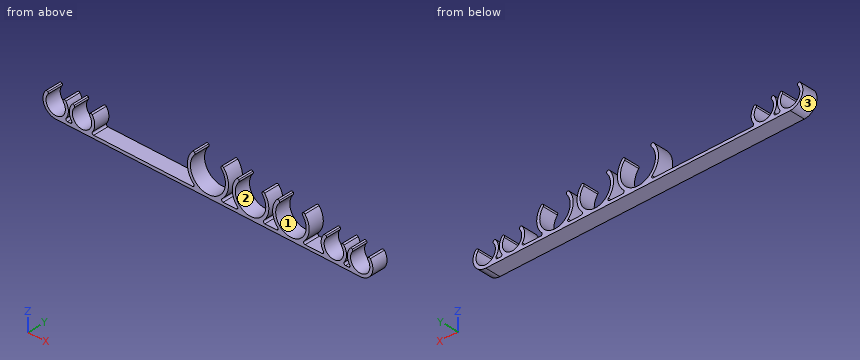
```python
from build123d import *

# Parameters (mm, degrees)
F1_DEPTH = 10


with BuildPart() as f1:
    # F0 (on Front) → F1 (new body)
    with BuildSketch(Plane.XZ):
        with BuildLine():
            Line((-100, 0), (0, 0))
            Line((0, 0), (100, 0))
            ThreePointArc((100, 0), (107.478558, 4.636017), (106.652751, 13.396128))
            ThreePointArc((106.652751, 13.396128), (105.9242, 13.789474), (105.148908, 13.498908))
            ThreePointArc((105.148908, 13.498908), (104.858342, 12.859987), (105.059278, 12.187474))
            ThreePointArc((105.059278, 12.187474), (100, 2), (94.940722, 12.187474))
            ThreePointArc((94.940722, 12.187474), (95.141658, 12.859987), (94.851092, 13.498908))
            ThreePointArc((94.851092, 13.498908), (94.0758, 13.789474), (93.347249, 13.396128))
            ThreePointArc((93.347249, 13.396128), (91.651649, 8.515919), (93.152004, 3.572193))
            ThreePointArc((93.152004, 3.572193), (93.218505, 2.537503), (92.331884, 2))
            Line((92.331884, 2), (90.368116, 2))
            ThreePointArc((90.368116, 2), (89.481495, 2.537503), (89.547996, 3.572193))
            ThreePointArc((89.547996, 3.572193), (91.048351, 8.515919), (89.352751, 13.396128))
            ThreePointArc((89.352751, 13.396128), (88.6242, 13.789474), (87.848908, 13.498908))
            ThreePointArc((87.848908, 13.498908), (87.558342, 12.859987), (87.759278, 12.187474))
            ThreePointArc((87.759278, 12.187474), (82.7, 2), (77.640722, 12.187474))
            ThreePointArc((77.640722, 12.187474), (77.841658, 12.859987), (77.551092, 13.498908))
            ThreePointArc((77.551092, 13.498908), (76.7758, 13.789474), (76.047249, 13.396128))
            ThreePointArc((76.047249, 13.396128), (74.351649, 8.515919), (75.852004, 3.572193))
            ThreePointArc((75.852004, 3.572193), (75.918505, 2.537503), (75.031884, 2))
            Line((75.031884, 2), (63.880832, 2))
            ThreePointArc((63.880832, 2), (62.960965, 2.607768), (63.159229, 3.692308))
            ThreePointArc((63.159229, 3.692308), (66.492584, 11.578174), (63.721535, 19.678756))
            ThreePointArc((63.721535, 19.678756), (62.998575, 20.037824), (62.245967, 19.745967))
            ThreePointArc((62.245967, 19.745967), (61.954109, 19.084362), (62.184612, 18.398964))
            ThreePointArc((62.184612, 18.398964), (54.5, 2), (46.815388, 18.398964))
            ThreePointArc((46.815388, 18.398964), (47.045891, 19.084362), (46.754033, 19.745967))
            ThreePointArc((46.754033, 19.745967), (46.001425, 20.037824), (45.278465, 19.678756))
            ThreePointArc((45.278465, 19.678756), (42.507416, 11.578174), (45.840771, 3.692308))
            ThreePointArc((45.840771, 3.692308), (46.039035, 2.607768), (45.119168, 2))
            Line((45.119168, 2), (37.380832, 2))
            ThreePointArc((37.380832, 2), (36.460965, 2.607768), (36.659229, 3.692308))
            ThreePointArc((36.659229, 3.692308), (39.992584, 11.578174), (37.221535, 19.678756))
            ThreePointArc((37.221535, 19.678756), (36.498575, 20.037824), (35.745967, 19.745967))
            ThreePointArc((35.745967, 19.745967), (35.454109, 19.084362), (35.684612, 18.398964))
            ThreePointArc((35.684612, 18.398964), (28, 2), (20.315388, 18.398964))
            ThreePointArc((20.315388, 18.398964), (20.545891, 19.084362), (20.254033, 19.745967))
            ThreePointArc((20.254033, 19.745967), (19.501425, 20.037824), (18.778465, 19.678756))
            ThreePointArc((18.778465, 19.678756), (16.007416, 11.578174), (19.340771, 3.692308))
            ThreePointArc((19.340771, 3.692308), (19.539035, 2.607768), (18.619168, 2))
            Line((18.619168, 2), (10, 2))
            ThreePointArc((10, 2), (9.071523, 2.628609), (9.310345, 3.724138))
            ThreePointArc((9.310345, 3.724138), (13.481586, 12.795141), (10.279021, 22.25167))
            ThreePointArc((10.279021, 22.25167), (9.557644, 22.602597), (8.810505, 22.310505))
            ThreePointArc((8.810505, 22.310505), (8.518413, 21.64343), (8.756203, 20.955126))
            ThreePointArc((8.756203, 20.955126), (0, 2), (-8.756203, 20.955126))
            ThreePointArc((-8.756203, 20.955126), (-8.518413, 21.64343), (-8.810505, 22.310505))
            ThreePointArc((-8.810505, 22.310505), (-9.557644, 22.602597), (-10.279021, 22.25167))
            ThreePointArc((-10.279021, 22.25167), (-13.481586, 12.795141), (-9.310345, 3.724138))
            ThreePointArc((-9.310345, 3.724138), (-9.071523, 2.628609), (-10, 2))
            Line((-10, 2), (-75.031884, 2))
            ThreePointArc((-75.031884, 2), (-75.918505, 2.537503), (-75.852004, 3.572193))
            ThreePointArc((-75.852004, 3.572193), (-74.351649, 8.515919), (-76.047249, 13.396128))
            ThreePointArc((-76.047249, 13.396128), (-76.7758, 13.789474), (-77.551092, 13.498908))
            ThreePointArc((-77.551092, 13.498908), (-77.841658, 12.859987), (-77.640722, 12.187474))
            ThreePointArc((-77.640722, 12.187474), (-82.693985, 2.000003), (-87.766539, 12.177883))
            ThreePointArc((-87.766539, 12.177883), (-87.566811, 12.84983), (-87.857312, 13.487806))
            ThreePointArc((-87.857312, 13.487806), (-88.63355, 13.778306), (-89.362299, 13.383515))
            ThreePointArc((-89.362299, 13.383515), (-91.048505, 8.508011), (-89.547996, 3.572193))
            ThreePointArc((-89.547996, 3.572193), (-89.481495, 2.537503), (-90.368116, 2))
            Line((-90.368116, 2), (-92.331884, 2))
            ThreePointArc((-92.331884, 2), (-93.218505, 2.537503), (-93.152004, 3.572193))
            ThreePointArc((-93.152004, 3.572193), (-91.651649, 8.515919), (-93.347249, 13.396128))
            ThreePointArc((-93.347249, 13.396128), (-94.0758, 13.789474), (-94.851092, 13.498908))
            ThreePointArc((-94.851092, 13.498908), (-95.141658, 12.859987), (-94.940722, 12.187474))
            ThreePointArc((-94.940722, 12.187474), (-100, 2), (-105.059278, 12.187474))
            ThreePointArc((-105.059278, 12.187474), (-104.858342, 12.859987), (-105.148908, 13.498908))
            ThreePointArc((-105.148908, 13.498908), (-105.9242, 13.789474), (-106.652751, 13.396128))
            ThreePointArc((-106.652751, 13.396128), (-107.478558, 4.636017), (-100, 0))
        make_face()
    extrude(amount=F1_DEPTH)


solid = f1.part
```
Source: CAD feature listing. Evaluate the final solid. Frame: model axes, mm. Face numbers are marked on the shaded views. Give positions to 0.01 mm unless a question says otherwise; leave off trailing zeros. Order: outer loops, then holes, each group sorted by start corner. A loop starts at its lowest first (then second) coordinate and runs counter-clockwise, first axis right, second up.
(1) Material intervals for line 1 along X through (y, z) = (-5.75, 17); line 2 along X through (y, z) = (-0.75, 15); line 3 along Z through (x, y) = (-24.5, -7), sorted ascending.
(2) Pull-direction query (Z, two-part tool) for the marked faces 1, 2 and 3; classes: +Z half, -Z half, draft (parallel to the pull), parting line (faces both ways), or undercut.
(3) Section query A-A (x = 28). Return the cut outline in (y, z), plus the area to 3 significant figures.
(4) Contact query for flat-ended pins moving along their axis: P1, Ø1, axis at y = -1, z = 20, coming from the -X side; P2, Ø1.6, axis at x = -91.5, y = -6, coming from the +Z side; P3, Ø10, axis at x = 100, z = 8.35, coming from the -Y side; P4, Ø2, axis at y = -6.5, z = 5.5, coming from the +X side. Output: stop coordinate, or through.
(5) Section query B-B (z = 9). State how many separate pieces and enclosed holes the cut face has, plus the area to 3 significant figures.
Outcome:
1. line 1: x = -13.04 to -10.95, 10.95 to 13.04, 17.09 to 19.34, 36.66 to 38.91, 43.59 to 45.84, 63.16 to 65.41
1. line 2: x = -13.42 to -11.4, 11.4 to 13.42, 16.38 to 18.46, 37.54 to 39.62, 42.88 to 44.96, 64.04 to 66.12
1. line 3: z = 0 to 2
2. face 1: undercut
2. face 2: undercut
2. face 3: parting line
3. outline: (-10, 0) - (0, 0) - (0, 2) - (-10, 2) - close
3. area: 20.0 mm2
4. P1: stops at x = -12.09
4. P2: stops at z = 11.58
4. P3: passes through
4. P4: stops at x = 108.14
5. separate pieces: 14
5. enclosed holes: 0
5. area: 287 mm2
